Could you check a few things on this model? Use its own coordinates, in mm. Round coordinates to 2 decimals unless told otherwise and drop trailing zeros. Write each loop counter-clockwise with the first axis right and the second up, starting at its lowest first coordinate (ties: lowest second). Pieces come first, ordered by that corner, then holes. Notation, with made-up numbers: (15.5, 2) -> (44.5, 2) arc R15 cw to (44.5, 10) -> close; hole circle Ø11 at (47, 13.5). An arc over 180 degrees is marked (long way). Answer as CSV lines item,"result". Start each with the question number.
Q1. If I drill on line 1 (Z direction, x = 24, y = -3); line 2 (Z direction, x = 17.5, y = -7.5); line 3 (Z direction, x = -49.5, y = -3), over which ranges is the centre line in solid material (lowest first)? Write a range as [from, to].
Q2. Imagine slicing it at A-A on z = -54.5. Please give me the cut outline in (x, y), and give its area (3 significant figures).
Q3. Imagine slicing it at B-B on y = -6.5. Give the number of separate pieces and of enclosed holes in the cut face, and give its area (3 significant figures).
Q4. Will this pin go through, and if not, where does the flat tip stop? pin 1 Ø3.5 at (x, z) = (-24, 17) entering from +Y.
Q5. If we mould it in two halves opening along X, with no side actions, what happens to faces 1 (the flat face through (-1, -5, -77)), 2 (the flat face through (-55, -5, 39)), 3 (the cylindrical face through (-24, -5, 19))? For each: pulls with the +X half, pulls with the -X half, needs draft (parallel to the pull), parting line crosses it, or undercut.
from build123d import *

# Parameters (mm, degrees)
F0_W      = 110
F0_H      = 94
F1_DEPTH  = 10
F2_R      = 2
F3_DEPTH  = 25
F4_W      = 110
F4_H      = 111
F4_H_2    = 15
F5_DEPTH  = 10
F6_R      = 2.5
F7_DEPTH  = 25
F8_W      = 110
F8_H      = 15
F9_DEPTH  = 10
F10_R     = 2.5
F11_DEPTH = 25


with BuildPart() as f1:
    # F0 (on Front) → F1 (new body)
    with BuildSketch(Plane.XZ):
        Rectangle(F0_W, F0_H)
    extrude(amount=F1_DEPTH)

    # F2 (on face) → F3 (cut)
    with BuildSketch(Plane.XZ.offset(10)):
        with Locations((-46, 43)):
            Circle(F2_R)
        with Locations((-24, 43)):
            Circle(F2_R)
        with Locations((-46, 17)):
            Circle(F2_R)
        with Locations((-24, 17)):
            Circle(F2_R)
        with Locations((46, 43)):
            Circle(F2_R)
        with Locations((24, 43)):
            Circle(F2_R)
        with Locations((24, 17)):
            Circle(F2_R)
        with Locations((46, 17)):
            Circle(F2_R)
        with Locations((-46, -17)):
            Circle(F2_R)
        with Locations((-46, -43)):
            Circle(F2_R)
        with Locations((-24, -43)):
            Circle(F2_R)
        with Locations((-24, -17)):
            Circle(F2_R)
        with Locations((24, -17)):
            Circle(F2_R)
        with Locations((24, -43)):
            Circle(F2_R)
        with Locations((46, -43)):
            Circle(F2_R)
        with Locations((46, -17)):
            Circle(F2_R)
    extrude(amount=-F3_DEPTH, mode=Mode.SUBTRACT)

    # F4 (on Front) → F5 (join)
    with BuildSketch(Plane.XZ):
        with Locations((0, 102.5)):
            Rectangle(F4_W, F4_H)
        with Locations((0, -54.5)):
            Rectangle(F4_W, F4_H_2)
    extrude(amount=F5_DEPTH)

    # F6 (on face) → F7 (cut)
    with BuildSketch(Plane.XZ.offset(10)):
        with Locations((-47.5, -54.5)):
            Circle(F6_R)
        with Locations((-17.5, -54.5)):
            Circle(F6_R)
        with Locations((17.5, -54.5)):
            Circle(F6_R)
        with Locations((47.5, -54.5)):
            Circle(F6_R)
        with Locations((-47.5, 150.5)):
            Circle(F6_R)
        with Locations((-17.5, 150.5)):
            Circle(F6_R)
        with Locations((17.5, 150.5)):
            Circle(F6_R)
        with Locations((47.5, 150.5)):
            Circle(F6_R)
    extrude(amount=-F7_DEPTH, mode=Mode.SUBTRACT)

    # F8 (on Front) → F9 (join)
    with BuildSketch(Plane.XZ):
        with Locations((0, -69.5)):
            Rectangle(F8_W, F8_H)
    extrude(amount=F9_DEPTH)

    # F10 (on face) → F11 (cut)
    with BuildSketch(Plane.XZ.offset(10)):
        with Locations((-21, -69)):
            Circle(F10_R)
        with Locations((21, -69)):
            Circle(F10_R)
    extrude(amount=-F11_DEPTH, mode=Mode.SUBTRACT)


solid = f1.part
Checks:
1,line 1,"[-77, -45], [-41, -19], [-15, 15], [19, 41], [45, 158]"
1,line 2,"[-77, -57], [-52, 148], [153, 158]"
1,line 3,"[-77, -56], [-53, 149], [152, 158]"
2,outline,"(-55, -10) -> (-50, -10) -> (-50, 0) -> (-55, 0) -> close; (-45, -10) -> (-20, -10) -> (-20, 0) -> (-45, 0) -> close; (-15, -10) -> (15, -10) -> (15, 0) -> (-15, 0) -> close; (20, -10) -> (45, -10) -> (45, 0) -> (20, 0) -> close; (50, -10) -> (55, -10) -> (55, 0) -> (50, 0) -> close"
2,area,"900 mm^2"
3,separate pieces,"1"
3,enclosed holes,"26"
3,area,"25,500 mm^2"
4,pin 1,"through"
5,face 1,"needs draft"
5,face 2,"pulls with the -X half"
5,face 3,"undercut"
